Input: part model. Units: mm. Frame: model coordinates. Give positions to 0.01 mm unless a question says otherwise; leave off trailing zeros. Loops run counter-clockwise (first coordinate to the right, second up) from the corner with the lowest first, then second, coordinate; pieces in that order, holes last. Notation, with made-up numbers: M 71,72 L 79,72 A30 cw 79,105 Z; hole C -40,4 d9. An arc over 180 degrees is marked long. Answer as a JSON object with one key per item and string values. Group by question number.
Autodesk Inventor part; units mm, degrees
ref_plane "YZ Plane" through (0, 0, 0) normal (1, 0, 0) x (0, 1, 0)
ref_plane "XZ Plane" through (0, 0, 0) normal (0, 1, 0) x (-1, 0, 0)
ref_plane "XY Plane" through (0, 0, 0) normal (0, 0, 1) x (1, 0, 0)
sketch "Sketch1" plane through (0, 0, 0) normal (0, 1, 0) x (-1, 0, 0)
  line L0 (-4.8543, -9.3666) -> (-103.2793, -9.3666)
  line L1 (-103.2793, -9.3666) -> (-103.2793, -423.7041)
  line L2 (-103.2793, -423.7041) -> (-4.8543, -423.7041)
  line L3 (-4.8543, -423.7041) -> (-4.8543, -9.3666)
  line L4 (-103.2793, -423.7041) -> (-89.8935, -423.7041) construction
  line L5 (-103.2793, -423.7041) -> (-89.8935, -423.7041) construction
  line L6 (-89.8935, -423.7041) -> (-89.8935, -403.6381) construction
  line L7 (-89.8935, -403.6381) -> (-89.8935, -351.0601)
  line L8 (-89.8935, -351.0601) -> (-89.8935, -342.5935) construction
  line L9 (-89.8935, -342.5935) -> (-89.8935, -290.0155)
  line L10 (-89.8935, -290.0155) -> (-89.8935, -281.5488) construction
  line L11 (-89.8935, -281.5488) -> (-89.8935, -228.9708)
  line L12 (-89.8935, -228.9708) -> (-89.8935, -220.5041) construction
  line L13 (-89.8935, -220.5041) -> (-89.8935, -167.9261)
  line L14 (-89.8935, -167.9261) -> (-89.8935, -159.4595) construction
  line L15 (-89.8935, -159.4595) -> (-89.8935, -106.8815)
  line L16 (-89.8935, -403.6381) -> (-17.2495, -403.6381)
  line L17 (-17.2495, -351.0601) -> (-89.8935, -351.0601)
  line L18 (-89.8935, -342.5935) -> (-17.2495, -342.5935)
  line L19 (-17.2495, -290.0155) -> (-89.8935, -290.0155)
  line L20 (-89.8935, -281.5488) -> (-17.2495, -281.5488)
  line L21 (-17.2495, -228.9708) -> (-89.8935, -228.9708)
  line L22 (-89.8935, -220.5041) -> (-17.2495, -220.5041)
  line L23 (-17.2495, -167.9261) -> (-89.8935, -167.9261)
  line L24 (-89.8935, -159.4595) -> (-17.2495, -159.4595)
  line L25 (-17.2495, -106.8815) -> (-89.8935, -106.8815)
  line L26 (-17.2495, -373.9201) -> (-21.8723, -377.3491)
  line L27 (-17.2495, -380.7781) -> (-21.8723, -377.3491)
  line L28 (-17.2495, -319.7335) -> (-21.8723, -316.3045)
  line L29 (-17.2495, -312.8755) -> (-21.8723, -316.3045)
  line L30 (-17.2495, -258.6888) -> (-21.8723, -255.2598)
  line L31 (-17.2495, -251.8308) -> (-21.8723, -255.2598)
  line L32 (-17.2495, -190.7861) -> (-21.8723, -194.2151)
  line L33 (-17.2495, -197.6441) -> (-21.8723, -194.2151)
  line L34 (-17.2495, -136.5995) -> (-21.8723, -133.1705)
  line L35 (-17.2495, -129.7415) -> (-21.8723, -133.1705)
  line L36 (-17.2495, -403.6381) -> (-17.2495, -380.7781)
  line L37 (-17.2495, -373.9201) -> (-17.2495, -351.0601)
  line L38 (-17.2495, -342.5935) -> (-17.2495, -319.7335)
  line L39 (-17.2495, -312.8755) -> (-17.2495, -290.0155)
  line L40 (-17.2495, -281.5488) -> (-17.2495, -258.6888)
  line L41 (-17.2495, -251.8308) -> (-17.2495, -228.9708)
  line L42 (-17.2495, -220.5041) -> (-17.2495, -197.6441)
  line L43 (-17.2495, -190.7861) -> (-17.2495, -167.9261)
  line L44 (-17.2495, -159.4595) -> (-17.2495, -136.5995)
  line L45 (-17.2495, -129.7415) -> (-17.2495, -106.8815)
  point P0 (0, 0)
  dimension "d0" = 98.425
  dimension "d1" = 414.3375
  dimension "d2" = 13.3858
  dimension "d4" = 20.066
  dimension "d5" = 52.578
  dimension "d6" = 8.4667
  dimension "d7" = 52.578
  dimension "d8" = 8.4667
  dimension "d9" = 52.578
  dimension "d10" = 8.4667
  dimension "d11" = 52.578
  dimension "d12" = 8.4667
  dimension "d13" = 52.578
  dimension "d16" = 72.644
extrude "Extrusion1" add sketch "Sketch1" along normal blind 2.8956
fillet "Fillet1" radius 2.54 20 edges at (17.2495, 1.4478, -106.8815) (17.2495, 1.4478, -159.4595) (17.2495, 1.4478, -167.9261) (17.2495, 1.4478, -228.9708) (17.2495, 1.4478, -290.0155) (17.2495, 1.4478, -351.0601) (17.2495, 1.4478, -403.6381) (17.2495, 1.4478, -342.5935) (17.2495, 1.4478, -281.5488) (17.2495, 1.4478, -220.5041) (89.8935, 1.4478, -403.6381) (89.8935, 1.4478, -342.5935) (89.8935, 1.4478, -281.5488) (89.8935, 1.4478, -220.5041) (89.8935, 1.4478, -159.4595) (89.8935, 1.4478, -106.8815) (89.8935, 1.4478, -167.9261) (89.8935, 1.4478, -228.9708) (89.8935, 1.4478, -290.0155) (89.8935, 1.4478, -351.0601)
fillet "Fillet2" radius 7.62 4 edges at (4.8543, 1.4478, -9.3666) (103.2793, 1.4478, -9.3666) (4.8543, 1.4478, -423.7041) (103.2793, 1.4478, -423.7041)
properties part number "clock face"
1. Material intervals for L1, parallel to Z at x = 83, y = 2.3; L2, parallel to X at y = 2.25, z = -127; L3, parallel to X at y = 1.9, z = -169.5, sorted ascending.
2. Mould query, pull axis X, two halves, no side actions, for faces 1 (the flat face through (54.8, 0, -167.6)), 2 (the cylindrical face through (101.11, 1.47, -421.41)), 3 (the cylindrical face through (7.146, 1.468, -421.531)). Classes: pulls with the +X half, pulls with the -X half, needs draft (parallel to the pull), parting line crosses it, or undercut.
3. First-contact query: P1, Ø8, axis at x = 84.5, z = -307, coming from the +Y side. Flat tip, straight axial feed; report the tip coordinate or a pass-through.
4. Section B-B (x = 76). Output: boundary loops of the cut face in (y, z), then the cut area to 3 significant figures.
5. Section C-C (y = 2.45). Count the separate pieces of the cut face and the enclosed holes in it, then the cut area to 3 significant figures.
6. Section A-A (z = -209.5). Output: boundary loops of the cut face in (x, y), then the cut area to 3 significant figures.
Geometry results:
{
 "1": {"L1": "-423.7 to -403.64, -351.06 to -342.59, -290.02 to -281.55, -228.97 to -220.5, -167.93 to -159.46, -106.88 to -9.37", "L2": "4.85 to 17.25, 89.89 to 103.28", "L3": "4.85 to 17.44, 89.7 to 103.28"},
 "2": {"face 1": "needs draft", "face 2": "pulls with the +X half", "face 3": "pulls with the -X half"},
 "3": {"P1": "through"},
 "4": {"outline": "M 0,-423.7 L 2.9,-423.7 L 2.9,-403.64 L 0,-403.64 Z; M 0,-351.06 L 2.9,-351.06 L 2.9,-342.59 L 0,-342.59 Z; M 0,-290.02 L 2.9,-290.02 L 2.9,-281.55 L 0,-281.55 Z; M 0,-228.97 L 2.9,-228.97 L 2.9,-220.5 L 0,-220.5 Z; M 0,-167.93 L 2.9,-167.93 L 2.9,-159.46 L 0,-159.46 Z; M 0,-106.88 L 2.9,-106.88 L 2.9,-9.37 L 0,-9.37 Z", "area": "439 mm2"},
 "5": {"separate pieces": "1", "enclosed holes": "5", "area": "21,700 mm2"},
 "6": {"outline": "M 4.85,0 L 17.25,0 L 17.25,2.9 L 4.85,2.9 Z; M 89.89,0 L 103.28,0 L 103.28,2.9 L 89.89,2.9 Z", "area": "74.7 mm2"}
}
